Can you work these out from the model? Positions are in its coordinate system, mm. A direction names the side the tool comes from. Give positions to 0.01 mm unless a question says otherwise; leave off trailing zeros. Order: outer loops, then holes, each group sorted by start corner. A loop starts at its lowest first (then second) coordinate and runs counter-clockwise, first axis right, second up. Notation, with made-up numbers: (5.25, -8.5) - (60.25, -8.5) arc R21 ccw to (60.25, 7.5) - close; hole circle Ø9 at (-21.5, -38.5). An arc over 180 degrees is marked (long way). Return JSON: item names as keys, results as strings.
```python
from build123d import *

# Parameters (mm, degrees)
F0_W      = 15.875
F0_H      = 47.752
F1_DEPTH  = 4.7625
F2_R      = 2.4511
F3_DEPTH  = 1.778
F4_W      = 13.589
F4_H      = 45.466
F4_R      = 3.2385
F5_DEPTH  = 8.382
F8_R      = 2.4765
F7_R      = 2.4765
F6_R      = 2.4765
F9_R      = 2.4765
F10_R     = 2.4765
F11_DEPTH = 8.382


with BuildPart() as f1:
    # F0 (on Top) → F1 (new body, symmetric)
    with BuildSketch(Plane.XY):
        Rectangle(F0_W, F0_H)
    extrude(amount=F1_DEPTH, both=True)

    # F2 (on face) → F3 (join)
    with BuildSketch(Plane.XY.offset(4.7625)):
        with Locations((-4.0132, 19.9517)):
            Circle(F2_R)
        with Locations((4.0132, 19.9517)):
            Circle(F2_R)
        with Locations((-4.0132, 11.9761)):
            Circle(F2_R)
        with Locations((4.0132, 11.9761)):
            Circle(F2_R)
        with Locations((4.0132, 4.0005)):
            Circle(F2_R)
        with Locations((-4.0132, 4.0005)):
            Circle(F2_R)
        with Locations((-4.0132, -4.0005)):
            Circle(F2_R)
        with Locations((4.0132, -4.0005)):
            Circle(F2_R)
        with Locations((4.0132, -11.9761)):
            Circle(F2_R)
        with Locations((-4.0132, -11.9761)):
            Circle(F2_R)
        with Locations((-4.0132, -19.9517)):
            Circle(F2_R)
        with Locations((4.0132, -19.9517)):
            Circle(F2_R)
    extrude(amount=F3_DEPTH)

    # F4 (on face) → F5 (cut)
    with BuildSketch(Plane(origin=(0, 0, -4.7625), x_dir=(1, 0, 0), z_dir=(0, 0, -1))):
        Rectangle(F4_W, F4_H)
        with Locations((0, -15.9512)):
            Circle(F4_R, mode=Mode.SUBTRACT)
        with Locations((0, -7.9756)):
            Circle(F4_R, mode=Mode.SUBTRACT)
        Circle(F4_R, mode=Mode.SUBTRACT)
        with Locations((0, 7.9756)):
            Circle(F4_R, mode=Mode.SUBTRACT)
        with Locations((0, 15.9512)):
            Circle(F4_R, mode=Mode.SUBTRACT)
    extrude(amount=-F5_DEPTH, mode=Mode.SUBTRACT)

    # F8 (on face) + F7 (on face) + F6 (on face) + F9 (on face) + F10 (on face) → F11 (cut)
    with BuildSketch(Plane(origin=(0, 0, -4.7625), x_dir=(1, 0, 0), z_dir=(0, 0, -1))):
        with Locations((0, 15.9512)):
            Circle(F8_R)
    with BuildSketch(Plane(origin=(0, 0, -4.7625), x_dir=(1, 0, 0), z_dir=(0, 0, -1))):
        with Locations((0, 7.9756)):
            Circle(F7_R)
    with BuildSketch(Plane(origin=(0, 0, -4.7625), x_dir=(1, 0, 0), z_dir=(0, 0, -1))):
        Circle(F6_R)
    with BuildSketch(Plane(origin=(0, 0, -4.7625), x_dir=(1, 0, 0), z_dir=(0, 0, -1))):
        with Locations((0, -7.9756)):
            Circle(F9_R)
    with BuildSketch(Plane(origin=(0, 0, -4.7625), x_dir=(1, 0, 0), z_dir=(0, 0, -1))):
        with Locations((0, -15.9512)):
            Circle(F10_R)
    extrude(amount=-F11_DEPTH, mode=Mode.SUBTRACT)


solid = f1.part
```
1. Thinking about a two-plate mould opening in Y: for faces 4 (the face through (7, 0, -4.762)), 5 (the face through (3.482, -22.345, 5.639)), which applies, +Y half, -Y half, draft (parallel to the pull), parting line (faces both ways), or undercut?
Checks:
{"face 4": "draft", "face 5": "undercut"}
2. Suppose I cut it at A-A (z = 3). State how many separate pieces and enclosed holes the cut face has, plus the area to 3 significant figures.
Checks:
{"separate pieces": "6", "enclosed holes": "6", "area": "209 mm^2"}
3. If I drill on L1, parallel to X at y = 2, z = -1; L2, parallel to Y at x = -6.75, z = -1; L3, parallel to X at y = -9.5, z = 0, over which ranges is the centre line in solid material (lowest first)? Write a range as [from, to].
Checks:
{"L1": "[-7.94, -6.79], [-2.55, -1.46], [1.46, 2.55], [6.79, 7.94]", "L2": "[-23.88, -22.73], [22.73, 23.88]", "L3": "[-7.94, -6.79], [-2.86, -1.95], [1.95, 2.86], [6.79, 7.94]"}
4. Suppose I cut it at B-B (y = 0). List the corners of the cut face in (x, z) for me.
Checks:
{"outline": "(-7.94, -4.76) - (-6.79, -4.76) - (-6.79, 3.62) - (-3.24, 3.62) - (-3.24, -4.76) - (-2.48, -4.76) - (-2.48, 3.62) - (2.48, 3.62) - (2.48, -4.76) - (3.24, -4.76) - (3.24, 3.62) - (6.79, 3.62) - (6.79, -4.76) - (7.94, -4.76) - (7.94, 4.76) - (-7.94, 4.76) - close"}
5. On a 3-axis mill with a long thin cutter (end or side, diameter ignored), from which of +Z, -Z, +X, -X, +Y, -Y can I reach the whole of each face in a straight line? I mean faces 1 (the face through (4, 12, 6.54)), 2 (the face through (-6.46, 4.11, 5.64)), 3 (the face through (0, 22.733, -1)). Say none if no direction works.
Checks:
{"face 1": "+Z, +X, -X, +Y, -Y", "face 2": "+Z", "face 3": "-Z"}
6. For pin 1 Ø5.5 at (x, y) = (-1, -16) entering from -Z; pin 2 Ø3 at (x, y) = (0, 0) entering from -Z; pin 3 Ø4.5 at (x, y) = (0, -15.95) entering from +Z, each with a flat end and sliding along its axis, tell me the tip position at first contact or that it passes through.
Checks:
{"pin 1": "z = -4.76", "pin 2": "z = 3.62", "pin 3": "z = 4.76"}
